Study the drawing (mm; zero at the part's minimum x, y, z) and answer. A direction names the side the tool comes from. Coordinates: 2 decimals unless noted, no trailing zeros. Loops run counter-clockwise (first coordinate to the right, second up) from the corner with the lowest first, then second, coordinate; pieces in that order, holes last. Notation, with made-up numbers: (-9.5, 83) -> (28.5, 83) arc R31 ccw to (28.5, 121) -> close; hole circle Ø9 at (56, 60.25). An arc over 180 degrees is marked (long way). One line per question, with ' | ' between items.
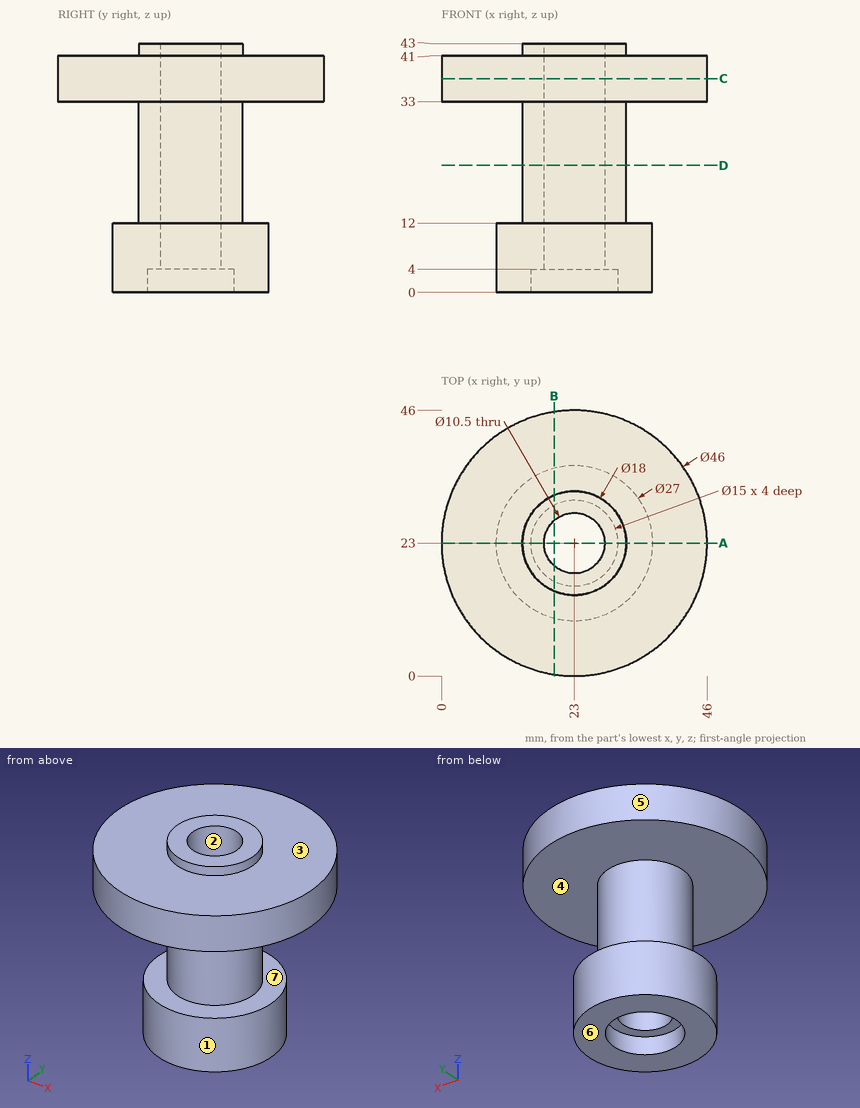
1) Find section B-B (x = 19.5). Write down the section's boundary in (y, z), plus the area to 3 significant figures.
Check values:
outline: (0.27, 33) -> (14.71, 33) -> (14.71, 12) -> (9.96, 12) -> (9.96, 0) -> (16.37, 0) -> (16.37, 4) -> (19.09, 4) -> (19.09, 43) -> (14.71, 43) -> (14.71, 41) -> (0.27, 41) -> close; (26.91, 4) -> (29.63, 4) -> (29.63, 0) -> (36.04, 0) -> (36.04, 12) -> (31.29, 12) -> (31.29, 33) -> (45.73, 33) -> (45.73, 41) -> (31.29, 41) -> (31.29, 43) -> (26.91, 43) -> close | area: 700 mm^2
2) Find the intervals of material crossed by line 1 along Y through (x, z) = (23, 1); line 2 along Z through (x, y) = (28, 31); line 3 along Z through (x, y) = (5, 14), in increasing order.
Check values:
line 1: y = 9.5 to 15.5, 30.5 to 36.5 | line 2: z = 0 to 12, 33 to 41 | line 3: z = 33 to 41
3) Flat-ended cylindrical pins translate along their axes: pin 1 (13.5 mm diameter, centred on x = 23, y = 23, fed in from -Z); pin 2 (5 mm diameter, centred on x = 10, z = 11, fed in from -Y); pin 3 (1 mm diameter, centred on x = 22, z = 14.5, fed in from -Y). Find the tip coordinate at first contact, or state that the pin passes through.
Check values:
pin 1: stops at z = 4 | pin 2: stops at y = 14.51 | pin 3: stops at y = 14.01
4) The mould has two halves that part along Z. Classify the marked faces 5, 6 and 7: released by +Z, released by -Z, zero draft, split by the parting line, or undercut.
Check values:
face 5: zero draft | face 6: released by -Z | face 7: undercut
5) For the marked faces 1, 2, 3 and 4, determine the directions among +Z, -Z, +X, -X, +Y, -Y from which every point of the face is accessible in a straight line to the end or side of a thin tool.
Check values:
face 1: -Z | face 2: +Z, -Z | face 3: +Z | face 4: none
6) Find section C-C (z = 37). Write down the section's boundary in (x, y).
Check values:
outline: circle Ø46 at (23, 23); hole circle Ø10.5 at (23, 23)
7) Find section A-A (y = 23). Write down the section's boundary in (x, z), plus the area to 4 significant figures.
Check values:
outline: (0, 33) -> (14, 33) -> (14, 12) -> (9.5, 12) -> (9.5, 0) -> (15.5, 0) -> (15.5, 4) -> (17.75, 4) -> (17.75, 43) -> (14, 43) -> (14, 41) -> (0, 41) -> close; (28.25, 4) -> (30.5, 4) -> (30.5, 0) -> (36.5, 0) -> (36.5, 12) -> (32, 12) -> (32, 33) -> (46, 33) -> (46, 41) -> (32, 41) -> (32, 43) -> (28.25, 43) -> close | area: 636.5 mm^2
8) Find section D-D (z = 22). Write down the section's boundary in (x, y).
Check values:
outline: circle Ø18 at (23, 23); hole circle Ø10.5 at (23, 23)
